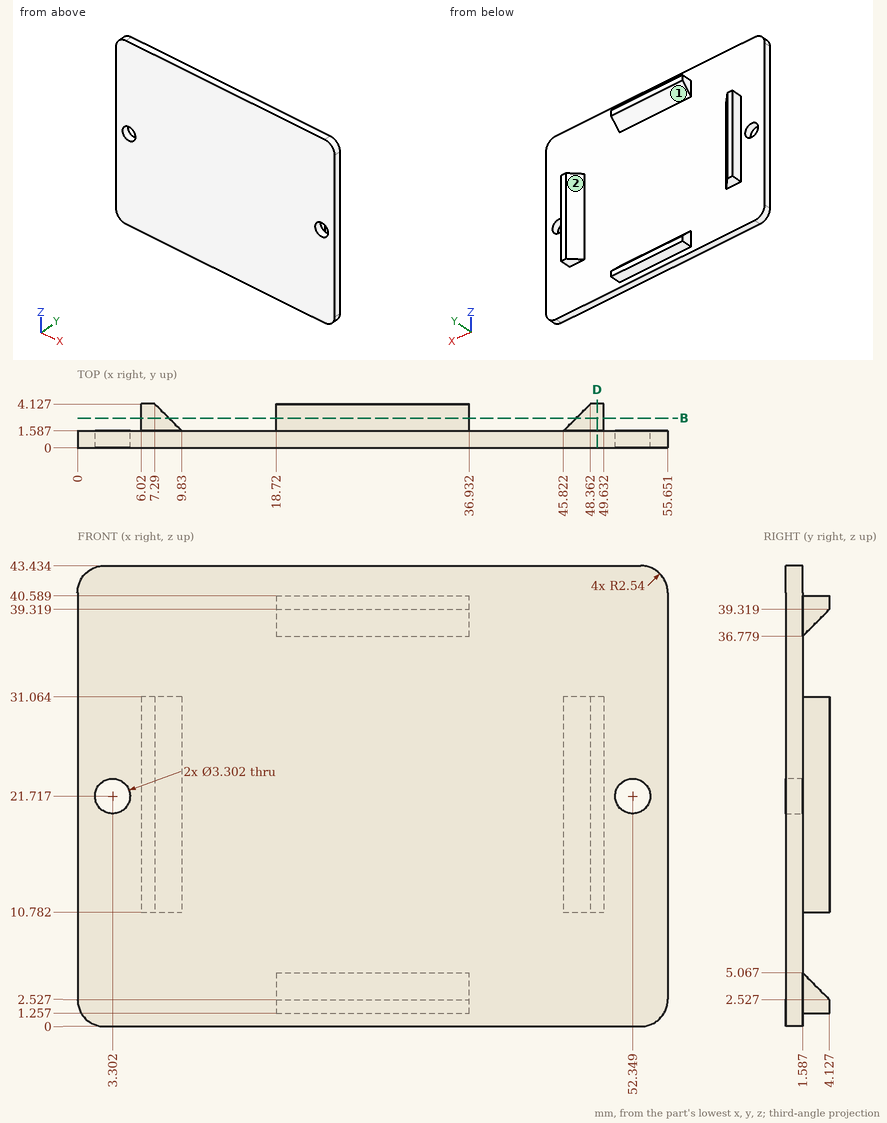
The drawing under review shows one solid part. Ordinate dimensions are in mm from its lowest x, y, z. Round coordinates to 2 decimals unless told otherwise and drop trailing zeros. Loops run counter-clockwise (first coordinate to the right, second up) from the corner with the lowest first, then second, coordinate; pieces in that order, holes last. Notation, with made-up numbers: M 12,71 L 38,71 A10 cw 38,81 Z; hole C -36,58.25 d5. An arc over 180 degrees is marked long. Answer as CSV lines item,"result". Start each with the question number.
Item 1: Mouldability with a two-part tool opening along X and no side actions: class the marked faces 1 and 2 as released by +X, released by -X, zero draft, split by the parting line, or undercut.
Item 2: Consider section D-D (x = 49). Write out the cut boundary in (y, z) (1 decimal).
Item 3: Wall thickness on line 1 (X direction, y = 1.65, z = 4); line 2 (Y direction, x = 29.5, z = 33.5); line 3 (Z direction, x = 32, y = 3.35) (1 decimal): over which ranges is each line inside the solid? List them lowest first. Write a range as [from, to].
Item 4: Insertion check: P1, Ø6, axis at x = 30, z = 11.5, coming from the +Y side; P2, Ø2, axis at x = 7.5, y = 3.5, coming from the +Z side; P3, Ø13, axis at x = 26.5, z = 31.5, coming from the +Y side. Each pin has a flat end and moves straight along its axis. Give the tip position at first contact, or say it passes through.
Item 5: Consider section B-B (y = 2.8). Write out the cut boundary in (x, z) (1 decimal), then the cut area to 3 significant figures.
Answer:
1,face 1,"zero draft"
1,face 2,"undercut"
2,outline,"M 0,0 L 1.6,0 L 1.6,10.8 L 4.1,10.8 L 4.1,31.1 L 1.6,31.1 L 1.6,43.4 L 0,43.4 Z"
3,line 1,"x = [18.72, 36.93]"
3,line 2,"y = [0, 1.59]"
3,line 3,"z = [1.3, 3.3], [38.5, 40.6]"
4,P1,"stops at y = 1.59"
4,P2,"stops at z = 31.06"
4,P3,"stops at y = 2.81"
5,outline,"M 6,10.8 L 8.6,10.8 L 8.6,31.1 L 6,31.1 Z; M 18.7,1.3 L 36.9,1.3 L 36.9,3.9 L 18.7,3.9 Z; M 18.7,38 L 36.9,38 L 36.9,40.6 L 18.7,40.6 Z; M 47,10.8 L 49.6,10.8 L 49.6,31.1 L 47,31.1 Z"
5,area,"200 mm^2"
